```python
from build123d import *

# Parameters (mm, degrees)
SKETCH1_W           = 95.25
SKETCH1_H           = 355.6
BOSS_EXTRUDE1_DEPTH = 6.35
SKETCH2_W           = 12.7
SKETCH2_H           = 12.7
CUT_EXTRUDE1_DEPTH  = 7.35
LPATTERN1_COUNT     = 16
LPATTERN1_PITCH     = 25.4
SKETCH3_W           = 12.7
SKETCH3_H           = 6.35
CUT_EXTRUDE2_DEPTH  = 7.35
LPATTERN4_COUNT     = 2
LPATTERN4_PITCH     = 76.2
SKETCH5_W           = 6.35
SKETCH5_H           = 254
BOSS_EXTRUDE2_DEPTH = 6.35
SKETCH6_W           = 6.35
SKETCH6_H           = 12.7
CUT_EXTRUDE3_DEPTH  = 7.35
SKETCH7_W           = 38.1
SKETCH7_H           = 6.35
BOSS_EXTRUDE4_DEPTH = 6.35
SKETCH8_W           = 12.7
SKETCH8_H           = 6.35
CUT_EXTRUDE4_DEPTH  = 7.35
SKETCH9_R           = 1.75
CUT_EXTRUDE5_DEPTH  = 7.35
SKETCH10_W          = 38.1
SKETCH10_H          = 114.8
CUT_EXTRUDE6_DEPTH  = 7.35
FILLET1_R           = 12.7


with BuildPart() as part:
    # Sketch1 → Boss-Extrude1 (new body)
    with BuildSketch(Plane.XY):
        with Locations((47.625, 177.8)):
            Rectangle(SKETCH1_W, SKETCH1_H)
    extrude(amount=BOSS_EXTRUDE1_DEPTH)

    # Sketch2 → Cut-Extrude1 (cut, through all)
    with BuildSketch(Plane.XY.offset(6.35)):
        with Locations((6.35, 6.35)):
            Rectangle(SKETCH2_W, SKETCH2_H)
        with Locations((88.9, 6.35)):
            Rectangle(SKETCH2_W, SKETCH2_H)
    cut_extrude1 = extrude(amount=-CUT_EXTRUDE1_DEPTH, mode=Mode.SUBTRACT)

    # LPattern1: Cut-Extrude1 ×16
    with Locations(*[(0, i * LPATTERN1_PITCH, 0) for i in range(1, LPATTERN1_COUNT)]):
        add(cut_extrude1, mode=Mode.SUBTRACT)

    # Sketch3 → Cut-Extrude2 (cut, through all)
    with BuildSketch(Plane.XY.offset(6.35)):
        with Locations((34.925, 41.275)):
            Rectangle(SKETCH3_W, SKETCH3_H)
        with Locations((60.325, 41.275)):
            Rectangle(SKETCH3_W, SKETCH3_H)
    cut_extrude2 = extrude(amount=-CUT_EXTRUDE2_DEPTH, mode=Mode.SUBTRACT)

    # LPattern4: Cut-Extrude2 ×2
    with Locations(*[(0, i * LPATTERN4_PITCH, 0) for i in range(1, LPATTERN4_COUNT)]):
        add(cut_extrude2, mode=Mode.SUBTRACT)

    # Sketch5 → Boss-Extrude2 (add, through all)
    with BuildSketch(Plane.XY.offset(6.35)):
        with Locations((9.525, 228.6)):
            Rectangle(SKETCH5_W, SKETCH5_H)
        with Locations((85.725, 228.6)):
            Rectangle(SKETCH5_W, SKETCH5_H)
    extrude(amount=-BOSS_EXTRUDE2_DEPTH)

    # Sketch6 → Cut-Extrude3 (cut, through all)
    with BuildSketch(Plane.XY.offset(6.35)):
        with Locations((3.175, 349.25)):
            Rectangle(SKETCH6_W, SKETCH6_H)
        with Locations((92.075, 349.25)):
            Rectangle(SKETCH6_W, SKETCH6_H)
    extrude(amount=-CUT_EXTRUDE3_DEPTH, mode=Mode.SUBTRACT)

    # Sketch7 → Boss-Extrude4 (add, through all)
    with BuildSketch(Plane.XY.offset(6.35)):
        with Locations((47.625, 117.475)):
            Rectangle(SKETCH7_W, SKETCH7_H)
    extrude(amount=-BOSS_EXTRUDE4_DEPTH)

    # Sketch8 → Cut-Extrude4 (cut, through all)
    with BuildSketch(Plane.XY.offset(6.35)):
        with Locations((34.925, 142.875)):
            Rectangle(SKETCH8_W, SKETCH8_H)
        with Locations((60.325, 142.875)):
            Rectangle(SKETCH8_W, SKETCH8_H)
    extrude(amount=-CUT_EXTRUDE4_DEPTH, mode=Mode.SUBTRACT)

    # Sketch9 → Cut-Extrude5 (cut, through all)
    with BuildSketch(Plane.XY.offset(6.35)):
        with Locations((12.7, 292.35)):
            Circle(SKETCH9_R)
        with Locations((12.7, 228.35)):
            Circle(SKETCH9_R)
    extrude(amount=-CUT_EXTRUDE5_DEPTH, mode=Mode.SUBTRACT)

    # Sketch10 → Cut-Extrude6 (cut, through all)
    with BuildSketch(Plane.XY.offset(6.35)):
        with Locations((38.1, 260.35)):
            Rectangle(SKETCH10_W, SKETCH10_H)
    extrude(amount=-CUT_EXTRUDE6_DEPTH, mode=Mode.SUBTRACT)

    # Fillet1
    fillet1_edges = [part.edges().sort_by_distance(p)[0] for p in [
        (19.05, 202.95, 3.175),
        (19.05, 317.75, 3.175),
        (57.15, 317.75, 3.175),
        (57.15, 202.95, 3.175),
    ]]
    fillet(fillet1_edges, radius=FILLET1_R)


solid = part.part
```
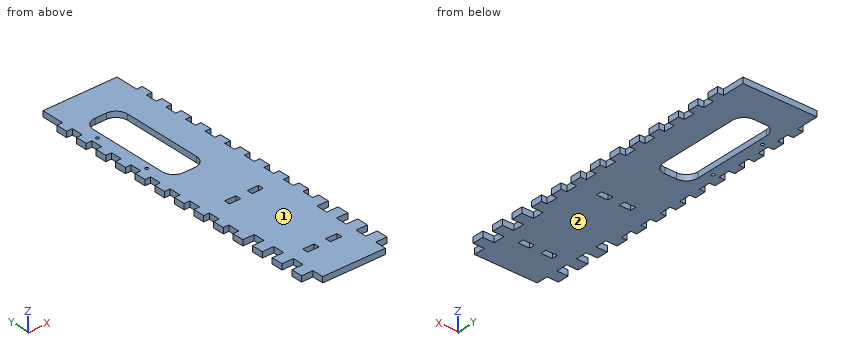
Build history of the part. All positions in model axes, mm. Face numbers are marked on the shaded views. Coordinates: 2 decimals unless noted, no trailing zeros. Order: outer loops, then holes, each group sorted by start corner. A loop starts at its lowest first (then second) coordinate and runs counter-clockwise, first axis right, second up.
Item 1: Drill centre lines: L1, parallel to X at y = 228.35, z = 5; L2, parallel to X at y = 43.5, z = 2.5 (3 decimals); L3, parallel to Y at x = 61, z = 4.5. Where is each one in solid material? Low to high.
Filled in:
L1: x = 0 to 10.95, 14.45 to 19.05, 57.15 to 95.25
L2: x = 0 to 28.575, 41.275 to 53.975, 66.675 to 95.25
L3: y = 0 to 38.1, 44.45 to 139.7, 146.05 to 355.6
Item 2: Mould opens along Z. For the marked faces 1 and 2 say: released by +Z, released by -Z, zero draft, split by the parting line, or undercut.
Filled in:
face 1: released by +Z
face 2: released by -Z
Item 3: Saw through at A-A on z = 5. State how many separate pieces and enclosed holes the cut face has, then the cut area to 3 significant figures.
Filled in:
separate pieces: 1
enclosed holes: 7
area: 26,200 mm2
Item 4: Drop flat-ended pins along their axis: pin 1 Ø1.9 at (x, z) = (92, 3.5) entering from -Y; pin 2 Ø3 at (y, z) = (131, 4.5) entering from -X; pin 3 Ø1.5 at (x, y) = (57.5, 55.5) entering from -Z; pin 4 Ø1.9 at (x, z) = (1.5, 4.5) entering from +Y. Give the stop position or say it passes through.
Filled in:
pin 1: stops at y = 12.7
pin 2: stops at x = 6.35
pin 3: stops at z = 0
pin 4: stops at y = 330.2
Item 5: Saw through at B-B on y = 183. List the corners of the cut face in (x, z).
Filled in:
outline: (6.35, 0) - (88.9, 0) - (88.9, 6.35) - (6.35, 6.35) - close
